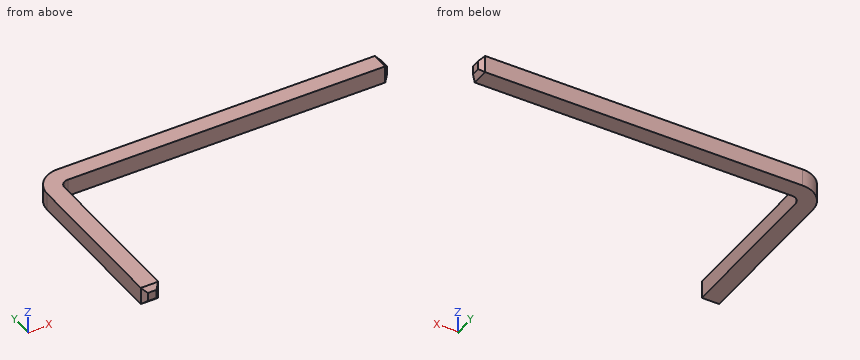
```python
from build123d import *

# Parameters (mm, degrees)
BODY_DEPTH     = 0.65
CHAMFER_2_SIZE = 0.1625


with BuildPart() as part:
    # Sketch1 → Body (new body)
    with BuildSketch(Plane.XY):
        with BuildLine():
            Line((0.95, 7), (13, 7))
            Line((13, 7), (13, 6.35))
            Line((13, 6.35), (0.95, 6.35))
            ThreePointArc((0.95, 6.35), (0.737867966, 6.262132034), (0.65, 6.05))
            Line((0.65, 6.05), (0.65, 0))
            Line((0.65, 0), (0, 0))
            Line((0, 0), (0, 6.05))
            ThreePointArc((0, 6.05), (0.278248558, 6.721751442), (0.95, 7))
        make_face()
    extrude(amount=BODY_DEPTH)

    # Chamfer 2
    chamfer_2_edges = [part.edges().sort_by_distance(p)[0] for p in [
        (13, 7, 0.325),
        (13, 6.35, 0.325),
        (13, 6.675, 0),
        (13, 6.675, 0.65),
        (0.65, 0, 0.325),
        (0, 0, 0.325),
        (0.325, 0, 0),
        (0.325, 0, 0.65),
    ]]
    chamfer(chamfer_2_edges, length=CHAMFER_2_SIZE)


solid = part.part
```
Design review of the part built by this model. Coordinates are the model's own, in mm. Coordinates: 2 decimals unless noted, no trailing zeros. Order: outer loops, then holes, each group sorted by start corner. A loop starts at its lowest first (then second) coordinate and runs counter-clockwise, first axis right, second up. Notation, with made-up numbers: M 55.25,-11.75 L 108.25,-11.75 A25 ccw 108.25,10.25 Z; hole C 28,-18 d7. An arc over 180 degrees is marked long. Answer as a JSON object with one key per item and string values. Group by question number.
1) Add section B-B, the plane x = 10.25. Write out the cut boundary in (y, z), then the cut area to 4 significant figures.
2) Add section A-A, the plane z = 0.3. Write out the cut boundary in (x, y).
3) Wall thickness on L1, parallel to X at y = 4.75, z = 0.25; L2, parallel to Y at x = 12.25, z = 0.25: over which ranges is each line inside the solid? List them lowest first.
4) For pin 1 (4 mm diameter, centred on x = 7, y = 6, fed in from -Z), flat-tipped, find the tip position at first contact; note if it passes through.
5) Add section C-C, the plane y = 2.75. Write out the cut boundary in (x, z), then the cut area to 4 significant figures.
Computed values:
{
 "1": {"outline": "M 6.35,0 L 7,0 L 7,0.65 L 6.35,0.65 Z", "area": "0.4225 mm^2"},
 "2": {"outline": "M 0,0.16 L 0.16,0 L 0.49,0 L 0.65,0.16 L 0.65,6.05 A0.3 cw 0.95,6.35 L 12.84,6.35 L 13,6.51 L 13,6.84 L 12.84,7 L 0.95,7 A0.95 ccw 0,6.05 Z"},
 "3": {"L1": "x = 0 to 0.65", "L2": "y = 6.35 to 7"},
 "4": {"pin 1": "stops at z = 0"},
 "5": {"outline": "M 0,0 L 0.65,0 L 0.65,0.65 L 0,0.65 Z", "area": "0.4225 mm^2"}
}
